Design review of the part built by this model. Coordinates are the model's own, in mm. A direction names the side the tool comes from. Round coordinates to 2 decimals unless told otherwise and drop trailing zeros. Write each loop counter-clockwise with the first axis right and the second up, starting at its lowest first coordinate (ties: lowest second). Pieces come first, ordered by that corner, then holes. Notation, with made-up numbers: (63, 52.5) - (117, 52.5) arc R35 ccw to (117, 90.5) - close; hole circle Ø11 at (77, -13). An arc over 180 degrees is marked (long way). Use one line per item in the form item = value.
```python
from build123d import *
from OCP.BRepFilletAPI import BRepFilletAPI_MakeChamfer

# Parameters (mm, degrees)
SKETCH_1_R             = 1.55
EXTRUDE_512_DEPTH      = 2.5
EXTRUDE_START          = 2.5
EXTRUDE_979_DEPTH      = 7.5
SKETCH_3_W             = 4.5
SKETCH_3_H             = 12.978713764
EXTRUDE_1_DEPTH        = 13.5
EXTRUDE_START_2        = -0.866441
EXTRUDE_2_DEPTH        = 12.978713764
SKETCH_5_R             = 1.55
CUT_EXTRUDE_1800_DEPTH = 36.225185951
CUT_EXTRUDE_START      = 9
SKETCH_5_3_R           = 1.55
CUT_EXTRUDE_1842_DEPTH = 2
CHAMFER_1_SIZE         = 0.615
CHAMFER_1_SIZE2        = 0.355070416
FILLET_5_R             = 0.75
FILLET_6_R             = 0.25
FILLET_8_R             = 1


with BuildPart() as part:
    # 草图1 → Extrude 512 (new body)
    with BuildSketch(Plane(origin=(0, 0, 0), x_dir=(1, 0, 0), z_dir=(0, 1, 0))):
        with BuildLine():
            Line((-10.1243866, 13.845154317), (6.15423406, 2.01804411))
            ThreePointArc((6.15423406, 2.01804411), (7.315700706, -5.315167685), (-0.017511089, -6.476634331))
            Line((-0.017511089, -6.476634331), (-10.1243866, 0.866440553))
            Line((-10.1243866, 0.866440553), (-10.1243866, 13.845154317))
        make_face()
        with Locations(Location((0, 0, 0), (0, 0, 270))):
            Circle(SKETCH_1_R, mode=Mode.SUBTRACT)
    extrude(amount=EXTRUDE_512_DEPTH)

    # 草图2 → Extrude 979 (add)
    with BuildSketch(Plane(origin=(0, 0, 0), x_dir=(1, 0, 0), z_dir=(0, 1, 0)).offset(EXTRUDE_START)):
        Polygon((-10.1243866, 0.866440553), (-0.017511089, -6.476634331), (-1.193081594, -8.09466832), (-11.299957105, -0.751593436), align=None)
        Polygon((7.329804565, 3.636078099), (-0.809505765, 9.549633202), (-1.98507627, 7.931599213), (6.15423406, 2.01804411), align=None)
    extrude(amount=-EXTRUDE_979_DEPTH)

    # 草图3 → 限位-1 (add)
    with BuildSketch(Plane(origin=(0, 0, 0), x_dir=(1, 0, 0), z_dir=(0, 1, 0))):
        with Locations((-12.3743866, 7.355797435)):
            Rectangle(SKETCH_3_W, SKETCH_3_H)
    extrude(amount=EXTRUDE_1_DEPTH)

    # 草图4 → 限位-2 (add)
    with BuildSketch(Plane.XY.offset(EXTRUDE_START_2)):
        Polygon((-14.6243866, 10.25), (-14.6243866, 13.5), (-21.1243866, 13.5), (-21.1243866, 1.5), (-17.6243866, 1.5), (-17.6243866, 10.25), align=None)
    extrude(amount=-EXTRUDE_2_DEPTH)

    # 草图5 → Cut-Extrude 1800 (cut, through all)
    with BuildSketch(Plane(origin=(-21.1243866, 0, 0), x_dir=(0, 0, -1), z_dir=(1, 0, 0))):
        with Locations(Location((7.355797435, 5.75, 0), (0, 0, 180))):
            Circle(SKETCH_5_R)
    extrude(amount=CUT_EXTRUDE_1800_DEPTH, mode=Mode.SUBTRACT)

    # 草图5<3> → Cut-Extrude 1842 (cut)
    with BuildSketch(Plane(origin=(-21.1243866, 0, 0), x_dir=(0, 0, -1), z_dir=(1, 0, 0)).offset(CUT_EXTRUDE_START)):
        Polygon((5.753650438, 2.975), (8.957944432, 2.975), (10.560091429, 5.75), (8.957944432, 8.525), (5.753650438, 8.525), (4.151503441, 5.75), align=None)
        with Locations(Location((7.355797435, 5.75, 0), (0, 0, 180))):
            Circle(SKETCH_5_3_R, mode=Mode.SUBTRACT)
    extrude(amount=CUT_EXTRUDE_1842_DEPTH, mode=Mode.SUBTRACT)

    # 倒角1: one chamfer whose edges measure the first distance from different faces: ONE call of the kernel's chamfer builder (chamfer() names one face for all edges)
    chamfer_1_edges_1 = [part.edges().sort_by_distance(p)[0] for p in [
        (0, 0, -1.55),
    ]]
    chamfer_1_side_1 = [part.faces().sort_by_distance(p)[0] for p in [
        (0, 1.25, -1.55),
    ]]
    chamfer_1_edges_2 = [part.edges().sort_by_distance(p)[0] for p in [
        (0, 2.5, -1.55),
    ]]
    chamfer_1_side_2 = [part.faces().sort_by_distance(p)[0] for p in [
        (-1.825655455, 2.5, -1.521026415),
    ]]
    chamfer_1_edges_3 = [part.edges().sort_by_distance(p)[0] for p in [
        (-21.1243866, 5.75, -8.905797435),
    ]]
    chamfer_1_side_3 = [part.faces().sort_by_distance(p)[0] for p in [
        (-19.3743866, 5.75, -8.905797435),
    ]]
    chamfer_1 = BRepFilletAPI_MakeChamfer(part.part.solid().wrapped)
    for e in chamfer_1_edges_1:
        chamfer_1.Add(CHAMFER_1_SIZE, CHAMFER_1_SIZE2, e.wrapped, chamfer_1_side_1[0].wrapped)  # the first distance lies on this face
    for e in chamfer_1_edges_2:
        chamfer_1.Add(CHAMFER_1_SIZE, CHAMFER_1_SIZE2, e.wrapped, chamfer_1_side_2[0].wrapped)  # the first distance lies on this face
    for e in chamfer_1_edges_3:
        chamfer_1.Add(CHAMFER_1_SIZE, CHAMFER_1_SIZE2, e.wrapped, chamfer_1_side_3[0].wrapped)  # the first distance lies on this face
    add(Compound.cast(chamfer_1.Shape()), mode=Mode.REPLACE)

    # 圆角5
    fillet_5_edges = [part.edges().sort_by_distance(p)[0] for p in [
        (-1.193081594, -1.25, 8.09466832),
        (-11.299957105, -1.25, 0.751593436),
        (-1.98507627, 1.25, -7.931599213),
        (-0.809505765, -1.25, -9.549633202),
        (7.329804565, -1.25, -3.636078099),
        (-0.017511089, 1.25, 6.476634331),
        (6.15423406, 1.25, -2.01804411),
    ]]
    fillet(fillet_5_edges, radius=FILLET_5_R)

    # 圆角6
    fillet_6_edges = [part.edges().sort_by_distance(p)[0] for p in [
        (-10.1243866, 1.25, -0.866440553),
    ]]
    fillet(fillet_6_edges, radius=FILLET_6_R)

    # 圆角8
    fillet_8_edges = [part.edges().sort_by_distance(p)[0] for p in [
        (-21.1243866, 7.5, -13.845154764),
        (-21.1243866, 7.5, -0.866441),
    ]]
    fillet(fillet_8_edges, radius=FILLET_8_R)


solid = part.part
```
Q1. Draft analysis for pull direction Y (two halves, no side actions). For faces 1 (the flat face through (-10.5, -1.2, -0.35)), 2 (the flat face through (-11.138, 7.157, -4.964)), 3 (the flat face through (-5.5, -5, 3.4)), state which applies: released by +Y, released by -Y, zero draft, split by the parting line, or undercut.
Calculated:
face_1 = zero draft
face_2 = undercut
face_3 = released by -Y
Q2. To check wall thickness, follow line 1 along X through (y, z) = (4.5, -12); line 2 along Z through (x, y) = (-18.9, 5.75); line 3 along X through (y, z) = (4, -5.75). State the ranges of each line that lie inside material, in increasing order. Write a range as from..to.
Calculated:
line_1 = -21.12..-17.62, -14.62..-10.12
line_2 = -13.85..-8.91, -5.81..-0.87
line_3 = -21.12..-17.62, -14.62..-12.12
Q3. For P1, Ø5, axis at x = -0.5, y = 1.5, coming from the -Z side; P2, Ø5, axis at x = -13.5, y = 9, coming from the +Z side; P3, Ø3, axis at x = 0, z = 0, coming from the -Y side; P4, Ø1, axis at x = -11.5, z = -7.5, coming from the -Y side, all flat-tipped, find the tip position at first contact; note any pin that passes through.
Calculated:
P1 = -9.25
P2 = -0.87
P3 = through
P4 = 0
Q4. We need section C-C on y = 12. Write out the cut boundary in (x, z).
Calculated:
outline = (-21.12, -12.85) arc R1 ccw to (-20.12, -13.85) - (-10.12, -13.85) - (-10.12, -0.87) - (-20.12, -0.87) arc R1 ccw to (-21.12, -1.87) - close
Q5. Machinability: for faces 4 (the flat face through (-3, 0, -3)), 5 (the flat face through (-1.613, -2.031, -8.444)), 6 (the flat face through (-16, 10.25, -7)), 7 (the flat face through (6.52, -2.03, -2.52)), 8 (the flat face through (-12.124, 5, -9)), which of the approach directions +Z, -Z, +X, -X, +Y, -Y give a long, thin tool a straight path to every point of the face, cutting with its end or side? Answer none if there is none.
Calculated:
face_4 = -Y
face_5 = -Z, -Y
face_6 = +Z, -Z, -Y
face_7 = +X, -Y
face_8 = +X
Q6. We need section A-A on y = 9.5. Write out the cut boundary in (x, z).
Calculated:
outline = (-21.12, -12.85) arc R1 ccw to (-20.12, -13.85) - (-17.62, -13.85) - (-17.62, -0.87) - (-20.12, -0.87) arc R1 ccw to (-21.12, -1.87) - close; (-14.62, -13.85) - (-10.12, -13.85) - (-10.12, -0.87) - (-14.62, -0.87) - close
Q7. We need section B-B on x = -13.5. Write out the cut boundary in (y, z).
Calculated:
outline = (0, -13.85) - (13.5, -13.85) - (13.5, -0.87) - (0, -0.87) - close; hole circle Ø3.1 at (5.75, -7.36)
Q8. We need section D-D on z = 2.75. Write out the cut boundary in (x, y), then the cut area to 3 significant figures.
Calculated:
outline = (-8.55, -5) - (-5.15, -5) - (-5.15, 0) - (8.29, 0) - (8.29, 2.5) - (-8.55, 2.5) - close
area = 59.1 mm2
